from build123d import *

# Parameters (mm, degrees)
SKETCH1_R           = 15
SKETCH1_R_2         = 11.2
BOSS_EXTRUDE1_DEPTH = 16
SKETCH2_R           = 5.5
SKETCH2_R_2         = 3.5
BOSS_EXTRUDE2_DEPTH = 5
SKETCH3_R           = 3.5
BOSS_EXTRUDE3_DEPTH = 10
SKETCH4_R           = 5.5
SKETCH4_R_2         = 3.5
BOSS_EXTRUDE4_DEPTH = 1.2


with BuildPart() as part:
    # Sketch1 → Boss-Extrude1 (new body)
    with BuildSketch(Plane.XY):
        Circle(SKETCH1_R)
        Circle(SKETCH1_R_2, mode=Mode.SUBTRACT)
    extrude(amount=BOSS_EXTRUDE1_DEPTH)

    # Sketch2 → Boss-Extrude2 (add)
    # profile 1 of 3: a face of its own
    with BuildSketch(Plane.XY):
        with Locations((-21.217622393, 12.25)):
            Circle(SKETCH2_R)
        with Locations((-21.217622393, 12.25)):
            Circle(SKETCH2_R_2, mode=Mode.SUBTRACT)
    # profile 2 of 3: a face of its own
    with BuildSketch(Plane.XY):
        with BuildLine():
            ThreePointArc((13.624389704, 6.275030295), (10.26570525, 15.701128433), (5.5, 24.5))
            ThreePointArc((5.5, 24.5), (0, 19), (-5.5, 24.5))
            ThreePointArc((-5.5, 24.5), (-10.26570525, 15.701128433), (-13.624389704, 6.275030295))
            ThreePointArc((-13.624389704, 6.275030295), (0, 15), (13.624389704, 6.275030295))
        make_face()
    # profile 3 of 3: a face of its own
    with BuildSketch(Plane.XY):
        with Locations((0, 24.5)):
            Circle(SKETCH2_R)
        with Locations(Location((0, 24.5, 0), (0, 0, 180))):
            Circle(SKETCH2_R_2, mode=Mode.SUBTRACT)
    extrude(amount=BOSS_EXTRUDE2_DEPTH)


with BuildPart() as boss_extrude2_kept_piece:
    # of the separate pieces the step leaves, the one the design keeps (boss_extrude2_pieces_kept)
    add(part.part.solids().sort_by_distance((15, 0, 0))[0])

    # Sketch3 → Boss-Extrude3 (add)
    with BuildSketch(Plane(origin=(0, 0, 0), x_dir=(-1, 0, 0), z_dir=(0, 0, -1))):
        with BuildLine():
            ThreePointArc((15, 0), (0, -15), (-15, 0))
            ThreePointArc((-15, 0), (-13.36999277, -30.430498916), (-6, -60))
            ThreePointArc((-6, -60), (0, -66), (6, -60))
            ThreePointArc((6, -60), (13.36999277, -30.430498916), (15, 0))
        make_face()
        with Locations((0, -60)):
            Circle(SKETCH3_R, mode=Mode.SUBTRACT)
    extrude(amount=-BOSS_EXTRUDE3_DEPTH)

    # Sketch4 → Boss-Extrude4 (add)
    with BuildSketch(Plane.XY.offset(5)):
        with Locations((0, 24.5)):
            Circle(SKETCH4_R)
        with Locations(Location((0, 24.5, 0), (0, 0, 180))):
            Circle(SKETCH4_R_2, mode=Mode.SUBTRACT)
    extrude(amount=BOSS_EXTRUDE4_DEPTH)


solid = boss_extrude2_kept_piece.part
The model under review builds one solid part; all positions refer to its coordinate system, in mm. A direction names the side the tool comes from. Give positions to 0.01 mm unless a question says otherwise; leave off trailing zeros. Order: outer loops, then holes, each group sorted by start corner. A loop starts at its lowest first (then second) coordinate and runs counter-clockwise, first axis right, second up. Notation, with made-up numbers: M 71,-29.5 L 97,-29.5 A21 cw 97,0.5 Z; hole C 81.25,66.5 d4. An arc over 180 degrees is marked long. Answer in a Markdown table with one row per item. Add a question column.
1. Add section A-A on z = 2. State the section outline as (x, y) points, plus the area to 3 significant figures.
2. To check wall thickness, follow line 1 along Y through (x, z) = (0, 6); line 2 along Y through (x, z) = (0, 4.25); line 3 along Y through (x, z) = (0, 6.5). State the ranges of each line that lie inside material, in increasing order.
3. Add section B-B on x = 0. State the section outline as (y, z) points, plus the area to 3 significant figures.
4. For pin 1 Ø5 at (x, z) = (11, 12) entering from +Y; pin 2 Ø15 at (x, y) = (0, -47.5) entering from +Z; pin 3 Ø5.5 at (x, y) = (0, 24.5) entering from +Z; pin 4 Ø9 at (x, y) = (1.5, 22) entering from +Z, all flat-tipped, find the tip position at first contact; note any pin that passes through.
5. Machinability: for faces 1 (the flat face through (4, 25, 6.2)), 2 (the cylindrical face through (10.323, 15.573, 2.465)), 3 (the cylindrical face through (-0.716, 29.953, 3.745)), which of the approach directions +Z, -Z, +X, -X, +Y, -Y give a long, thin tool a straight path to every point of the face, cutting with its end or side? Answer none if there is none.
6. Add section C-C on y = 1. State the section outline as (x, z) points.
7. Add section D-D on z = 12. State the section outline as (x, y) points, plus the area to 3 significant figures.
8. Mouldability with a two-part tool opening along X and no side actions: class faces 4 (the flat face through (0, 16, 5)), 5 (the cylindrical face through (-1.953, 14.872, 9.666)), 6 (the cylindrical face through (-1.615, -63.105, 4.93)) as released by +X, released by -X, zero draft, split by the parting line, or undercut.
The answers:
| question | item | result |
|---|---|---|
| 1 | outline | M -15,0 A160 ccw -6,-60 A6 ccw 6,-60 A160 ccw 15,0 A15 ccw 13.62,6.28 A65 ccw 5.5,24.5 A5.5 ccw -5.5,24.5 A65 ccw -13.62,6.28 A15 ccw Z; hole C 0,0 d22.4; hole C 0,-60 d7; hole C 0,24.5 d7 |
| 1 | area | 1,680 mm2 |
| 2 | line 1 | -66 to -63.5, -56.5 to -11.2, 11.2 to 15, 19 to 21, 28 to 30 |
| 2 | line 2 | -66 to -63.5, -56.5 to -11.2, 11.2 to 21, 28 to 30 |
| 2 | line 3 | -66 to -63.5, -56.5 to -11.2, 11.2 to 15 |
| 3 | outline | M -66,0 L -63.5,0 L -63.5,10 L -66,10 Z; M -56.5,0 L -11.2,0 L -11.2,16 L -15,16 L -15,10 L -56.5,10 Z; M 11.2,0 L 21,0 L 21,6.2 L 19,6.2 L 19,5 L 15,5 L 15,16 L 11.2,16 Z; M 28,0 L 30,0 L 30,6.2 L 28,6.2 Z |
| 3 | area | 606 mm2 |
| 4 | pin 1 | y = 12.36 |
| 4 | pin 2 | z = 10 |
| 4 | pin 3 | through |
| 4 | pin 4 | z = 6.2 |
| 5 | face 1 | +Z, +X, -X, +Y |
| 5 | face 2 | +Z, -Z, +X, +Y |
| 5 | face 3 | +Z |
| 6 | outline | M -14.97,0 L -11.16,0 L -11.16,16 L -14.97,16 Z; M 11.16,0 L 14.97,0 L 14.97,16 L 11.16,16 Z |
| 7 | outline | C 0,0 d30; hole C 0,0 d22.4 |
| 7 | area | 313 mm2 |
| 8 | face 4 | zero draft |
| 8 | face 5 | split by the parting line |
| 8 | face 6 | undercut |
